For this review, use the dimensioned drawing (mm, ordinates from the lowest corner) and the shaded views. Coordinates: 2 decimals unless noted, no trailing zeros. Loops run counter-clockwise (first coordinate to the right, second up) from the corner with the lowest first, then second, coordinate; pieces in that order, holes last. Notation, with made-up numbers: (55, 27) - (89, 27) arc R27 cw to (89, 50) - close; hole circle Ø1 at (-27, 41.5). An arc over 180 degrees is marked (long way). Answer in a Markdown table with one row per item. Add a question column.
(1) For P1, Ø2, axis at x = 2.465, y = 2.95, coming from the +Z side; P2, Ø1, axis at y = 4, z = 2.5, coming from the -X side, all flat-tipped, find the tip position at first contact; note any pin that passes through.
(2) We need section C-C on y = 1.55. Write out the cut boundary in (x, z), plus the area to 3 significant figures.
(3) We need section B-B on z = 1.25. Give the number of separate pieces and of enclosed holes in the cut face.
(4) Mouldability with a two-part tool opening along X and no side actions: class the marked faces 1, 2 and 3 as +X half, -X half, draft (parallel to the pull), parting line (faces both ways), or undercut.
(5) For line 1 along X through (y, z) = (3, 1.35) (1 decimal); line 2 along X through (y, z) = (1.8, 3.75) (1 decimal); line 3 along Y through (x, z) = (2.25, 2.8), list the stretches that pass through material, from the lowest coordinate up.
(6) We need section A-A on y = 2.95. Write out the cut boundary in (x, z) (1 decimal).
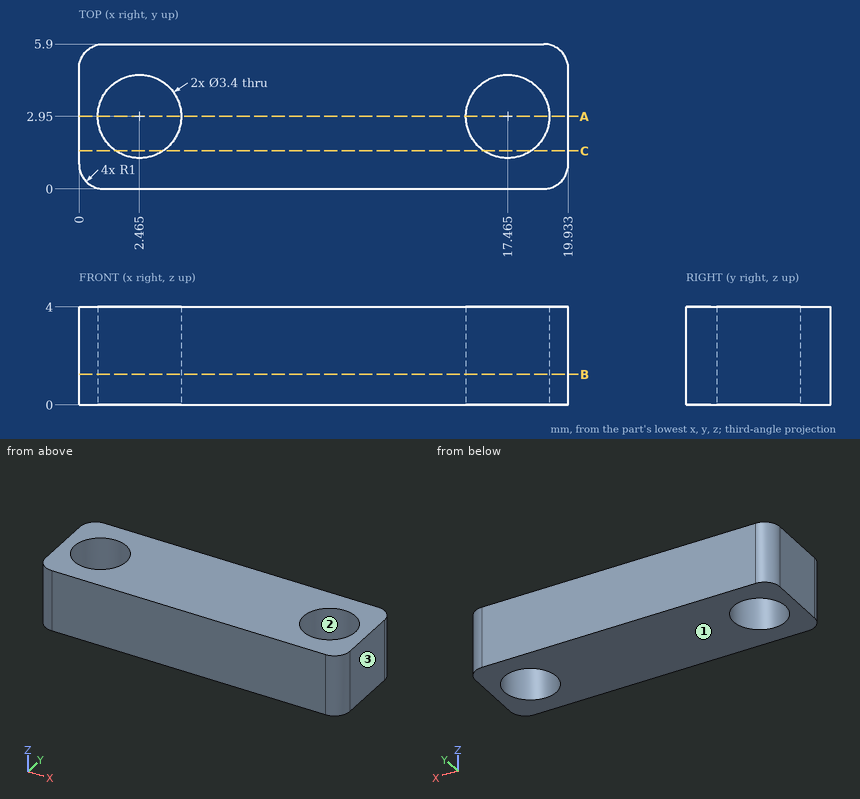
Outcome:
| question | item | result |
|---|---|---|
| 1 | P1 | through |
| 1 | P2 | x = 0 |
| 2 | outline | (0, 0) - (1.5, 0) - (1.5, 4) - (0, 4) - close; (3.43, 0) - (16.5, 0) - (16.5, 4) - (3.43, 4) - close; (18.43, 0) - (19.93, 0) - (19.93, 4) - (18.43, 4) - close |
| 2 | area | 64.3 mm² |
| 3 | separate pieces | 1 |
| 3 | enclosed holes | 2 |
| 4 | face 1 | draft |
| 4 | face 2 | undercut |
| 4 | face 3 | +X half |
| 5 | line 1 | 0 to 0.8, 4.2 to 15.8, 19.2 to 19.9 |
| 5 | line 2 | 0 to 1.2, 3.7 to 16.2, 18.7 to 19.9 |
| 5 | line 3 | 0 to 1.26, 4.64 to 5.9 |
| 6 | outline | (0, 0) - (0.8, 0) - (0.8, 4) - (0, 4) - close; (4.2, 0) - (15.8, 0) - (15.8, 4) - (4.2, 4) - close; (19.2, 0) - (19.9, 0) - (19.9, 4) - (19.2, 4) - close |
